Source: CAD feature listing. Evaluate the final solid. Frame: model axes, mm. A direction names the side the tool comes from. Round coordinates to 2 decimals unless told otherwise and drop trailing zeros. Loops run counter-clockwise (first coordinate to the right, second up) from the corner with the lowest first, then second, coordinate; pieces in that order, holes last. Notation, with made-up numbers: (56, 38) - (112, 38) arc R23 ccw to (112, 55) - close; hole circle Ø10 at (45, 81.5). An arc over 180 degrees is marked (long way). One line per question, with ' | ' between items. Start each with the question number.
1. Cut plane A-A (y = 0). Return loops of the section in (x, z), then the cut area to 3 significant figures.
2. Cut plane B-B (x = 1.65). Return loops of the section in (y, z), then the cut area to 3 significant figures.
3. Access query for faces 5 (the flat face through (3.5, 1, -12)), 6 (the flat face through (2.7, 3, -11)), 7 (the flat face through (2.7, -3, -11)). Directions: +Z, -Z, +X, -X, +Y, -Y. A direction counts if a zero-diameter tool reaches every point of the face in a straight line with its end or side. Return the directions, or none.
4. Pin query (flat end, axial travel): pin 1 (1.5 mm diameter, centred on x = 1, y = 1.5, fed in from +Z); pin 2 (4.5 mm diameter, centred on y = 0.5, z = -0.5, fed in from +X); pin 3 (1.6 mm diameter, centred on y = 0, z = 10.76, fed in from -X); pin 4 (1.5 mm diameter, centred on x = 1.5, y = 3.5, fed in from +Z). Return the tip coordinate at first contact, or that it passes through.
5. Mould query, pull axis Z, two halves, no side actions, for faces 1 (the cylindrical face through (2.996, 1.918, 9.962)), 2 (the flat face through (2.7, -3, 11)), 3 (the flat face through (0, 0, 0)), 4 (the cylindrical face through (1.479, -0.067, -15.694)). Classes: pulls with the +Z half, pulls with the -Z half, needs draft (parallel to the pull), parting line crosses it, or undercut.
6. Cut plane D-D (z = -2). Return loops of the section in (x, y).
7. Cut plane C-C (y = -3.5). Return loops of the section in (x, z), then the cut area to 4 significant figures.
8. Ray query, line 1 (Z direction, x = 0.35, y = -0.75); line 2 (X direction, y = 3, z = 3.5); line 3 (X direction, y = 4, z = 12.5). Return the intervals inside material, ascending.
```python
from build123d import *

# Parameters (mm, degrees)
F1_DEPTH = 3
F2_W     = 9.2
F2_H     = 3.976691
F3_DEPTH = 0.3
F4_R     = 2.07618
F5_DEPTH = 0.8
F6_R     = 0.2
F7_R     = 1
F8_DEPTH = 25


with BuildPart() as f1:
    # F0 (on Right) → F1 (new body)
    with BuildSketch(Plane.YZ):
        with BuildLine():
            Line((4.6, -14.5), (4.6, 14.5))
            ThreePointArc((4.6, 14.5), (0, 15.694247), (-4.6, 14.5))
            Line((-4.6, 14.5), (-4.6, -14.5))
            ThreePointArc((-4.6, -14.5), (0, -15.694247), (4.6, -14.5))
        make_face()
    extrude(amount=F1_DEPTH)

    # F2 (on face) → F3 (cut)
    with BuildSketch(Plane.YZ.offset(3)):
        with Locations((0, 10.756953)):
            Rectangle(F2_W, F2_H)
        with Locations((0, -10.756953)):
            Rectangle(F2_W, F2_H)
    extrude(amount=-F3_DEPTH, mode=Mode.SUBTRACT)

    # F4 (on face) → F5 (join)
    with BuildSketch(Plane.YZ.offset(2.7)):
        with Locations((0, 10.756953)):
            Circle(F4_R)
        with Locations((0, -10.756953)):
            Circle(F4_R)
    extrude(amount=F5_DEPTH)

    # F6
    f6_edges = [f1.edges().sort_by_distance(p)[0] for p in [
        (3.5, -2.07618, 10.756953),
        (3.5, -2.07618, -10.756953),
    ]]
    fillet(f6_edges, radius=F6_R)

    # F7 (on face) → F8 (cut)
    with BuildSketch(Plane.YZ.offset(3.5)):
        with Locations((0, 10.756953)):
            Circle(F7_R)
        with Locations((0, -10.756953)):
            Circle(F7_R)
    extrude(amount=-F8_DEPTH, mode=Mode.SUBTRACT)


solid = f1.part
```
Answers follow:
1) outline: (0, -15.69) - (3, -15.69) - (3, -12.83) - (3.3, -12.83) arc R0.2 ccw to (3.5, -12.63) - (3.5, -11.76) - (0, -11.76) - close; (0, -9.76) - (3.5, -9.76) - (3.5, -8.88) arc R0.2 ccw to (3.3, -8.68) - (3, -8.68) - (3, 8.68) - (3.3, 8.68) arc R0.2 ccw to (3.5, 8.88) - (3.5, 9.76) - (0, 9.76) - close; (0, 11.76) - (3.5, 11.76) - (3.5, 12.63) arc R0.2 ccw to (3.3, 12.83) - (3, 12.83) - (3, 15.69) - (0, 15.69) - close | area: 84.3 mm2
2) outline: (-4.6, -14.5) arc R9.46 ccw to (4.6, -14.5) - (4.6, 14.5) arc R9.46 ccw to (-4.6, 14.5) - close; hole circle Ø2 at (0, -10.76); hole circle Ø2 at (0, 10.76) | area: 275 mm2
3) face 5: +Z, -Z, +X, +Y, -Y | face 6: +X, +Y | face 7: +X, -Y
4) pin 1: stops at z = 15.66 | pin 2: stops at x = 3 | pin 3: passes through | pin 4: stops at z = 15.29
5) face 1: undercut | face 2: undercut | face 3: needs draft | face 4: pulls with the -Z half
6) outline: (0, -4.6) - (3, -4.6) - (3, 4.6) - (0, 4.6) - close
7) outline: (0, -15.02) - (3, -15.02) - (3, -12.75) - (2.7, -12.75) - (2.7, -8.77) - (3, -8.77) - (3, 8.77) - (2.7, 8.77) - (2.7, 12.75) - (3, 12.75) - (3, 15.02) - (0, 15.02) - close | area: 87.75 mm2
8) line 1: z = -15.66 to -11.42, -10.1 to 10.1, 11.42 to 15.66 | line 2: x = 0 to 3 | line 3: x = 0 to 2.7
